Autodesk Inventor part; units mm, degrees
ref_plane "YZ Plane" through (0, 0, 0) normal (1, 0, 0) x (0, 1, 0)
ref_plane "XZ Plane" through (0, 0, 0) normal (0, 1, 0) x (-1, 0, 0)
ref_plane "XY Plane" through (0, 0, 0) normal (0, 0, 1) x (1, 0, 0)
sketch "Sketch1" plane through (0, 0, 0) normal (0, 0, 1) x (1, 0, 0)
  line L0 (-9.0847, 275.4971) -> (0.0597, 261.7096)
  line L1 (0.0597, 261.7096) -> (-4.5238, 258.6697)
  line L2 (-4.5238, 258.6697) -> (-13.846, 272.7251)
  line L3 (-20.4878, 268.8466) -> (-13.846, 272.7251)
  line L4 (-9.0847, 275.4971) -> (-3.3614, 279.1755)
  line L5 (-20.4878, 268.8466) -> (-29.1232, 263.8039)
  line L6 (-3.3614, 279.1755) -> (5.4134, 283.9717)
  line L7 (11.2184, 194.7202) -> (22.61, 201.3724)
  line L8 (44.4638, 214.134) -> (54.3957, 219.9338)
  line L9 (4.4881, 206.2457) -> (-0.6932, 203.2201)
  line L10 (-0.6932, 203.2201) -> (-3.2145, 207.5378)
  line L11 (-3.2145, 207.5378) -> (1.9667, 210.5634)
  line L12 (-29.1232, 263.8039) -> (1.9667, 210.5634)
  line L13 (4.4881, 206.2457) -> (11.2184, 194.7202)
  line L14 (54.3957, 219.9338) -> (37.2403, 249.3118)
  line L15 (37.2403, 249.3118) -> (27.3211, 243.8901)
  line L16 (27.3211, 243.8901) -> (5.4134, 283.9717)
  line L17 (44.4638, 214.134) -> (22.61, 201.3724)
  point P0 (0, 0)
  dimension "d11" = 20
  dimension "d12" = 5.5
  dimension "d13" = 10
  dimension "d14" = 80
  dimension "d15" = 50
  dimension "d16" = 10
  dimension "d17" = 6
  dimension "d18" = 5
extrude "Extrusion1" add sketch "Sketch1" along normal blind 5.5
fillet "Fillet2" radius 8 2 edges at (37.2403, 249.3118, 2.75) (27.3211, 243.8901, 2.75)
fillet "Fillet3" radius 5 4 edges at (5.4134, 283.9717, 2.75) (54.3957, 219.9338, 2.75) (11.2184, 194.7202, 2.75) (-29.1232, 263.8039, 2.75)
properties part number "adelante"
The listing builds one solid part. Answer for the finished solid, in the listing's coordinates (mm). A direction names the side the tool comes from. Coordinates: 2 decimals unless noted, no trailing zeros. Order: outer loops, then holes, each group sorted by start corner. A loop starts at its lowest first (then second) coordinate and runs counter-clockwise, first axis right, second up. Notation, with made-up numbers: (27.5, -4.5) -> (69.5, -4.5) arc R15 ccw to (69.5, 17.5) -> close; hole circle Ø10 at (-22, 19.25). An arc over 180 degrees is marked (long way). Answer in a Markdown table with one row per item. Add a question column.
Item 1: Find the intervals of material crossed by L1, parallel to Y at x = -3.5, z = 3.7; L2, parallel to X at y = 218, z = 0.65; L3, parallel to X at y = 244, z = 0.9, in increasing order. Write a range as from..to.
Item 2: Each of these flat-tipped pins is pushed along its axis until it touches: P1, Ø1, axis at x = 30.5, z = 1.5, coming from the +Y side; P2, Ø2, axis at y = 210, z = 2, coming from the +X side; P3, Ø5, axis at x = 2, y = 258.5, coming from the -Z side; P4, Ø3, axis at y = 243, z = 0.5, coming from the +X side. Where does it stop, or does it pass through?
Item 3: Which of the six approach directions +Z, -Z, +X, -X, +Y, -Y give full straight-line access (tool end or side, diameter ignored) to faces 1 (the face through (-1.198, 280.358, 2.712)), 2 (the face through (-0.66, 209.03, 2.71)), 3 (the face through (-9.12, 265.6, 2.71)), 4 (the face through (6.563, 202.692, 2.712)), 5 (the face through (12, 240, 5.5))?
Item 4: Determine the mould class of faces 6 (the face through (52.38, 220.41, 2.79)), 7 (the face through (-4.577, 268.7, 2.712)), 8 (the face through (11.69, 196.74, 2.79)) for opening direction X: +X half, -X half, draft (parallel to the pull), parting line (faces both ways), or undercut.
Item 5: Find section B-B (x = 46.5). Write down the section's boundary in (y, z), then the cut area to 3 significant figures.
Item 6: Find section A-A (y = 254). Write down the section's boundary in (x, z), then the cut area to 3 significant figures.
Result set:
| question | item | result |
|---|---|---|
| 1 | L1 | y = 219.92..259.35, 267.08..279.09 |
| 1 | L2 | x = -2.38..50.89 |
| 1 | L3 | x = -17.56..40.12 |
| 2 | P1 | stops at y = 246.23 |
| 2 | P2 | stops at x = 39.1 |
| 2 | P3 | stops at z = 0 |
| 2 | P4 | stops at x = 41.8 |
| 3 | face 1 | +Z, -Z, -X, +Y |
| 3 | face 2 | +Z, -Z, -X |
| 3 | face 3 | +Z, -Z |
| 3 | face 4 | +Z, -Z, -Y |
| 3 | face 5 | +Z, +X, -X, +Y, -Y |
| 4 | face 6 | +X half |
| 4 | face 7 | undercut |
| 4 | face 8 | parting line |
| 5 | outline | (215.32, 0) -> (233.45, 0) -> (233.45, 5.5) -> (215.32, 5.5) -> close |
| 5 | area | 99.7 mm² |
| 6 | outline | (-23.4, 0) -> (21.8, 0) -> (21.8, 5.5) -> (-23.4, 5.5) -> close |
| 6 | area | 249 mm² |
